from build123d import *

# Parameters (mm, degrees)
BOSS_EXTRUDE1_DEPTH = 0.35
FILLET1_R           = 0.4
FILLET2_R           = 0.5
SKETCH4_W           = 8.5
SKETCH4_H           = 3.36
CUT_EXTRUDE1_DEPTH  = 0.115
SKETCH5_W           = 8.5
SKETCH5_H           = 3.36
CUT_EXTRUDE2_DEPTH  = 0.115
FILLET3_R           = 0.05
SKETCH8_W           = 7.02
SKETCH8_H           = 2.46
BOSS_EXTRUDE2_DEPTH = 0.005
SKETCH9_W           = 7.02
SKETCH9_H           = 2.46
BOSS_EXTRUDE3_DEPTH = 0.005
SKETCH10_W          = 0.5
SKETCH10_H          = 0.12
CUT_EXTRUDE3_DEPTH  = 0.005


with BuildPart() as part:
    # Sketch3 → Boss-Extrude1 (new body)
    with BuildSketch(Plane(origin=(0, 0, 0), x_dir=(1, 0, 0), z_dir=(0, 1, 0))):
        Polygon((-4.25, -4.25), (-3.17, -4.25), (-3.17, -11.79), (5.77, -11.79), (5.77, -7.61), (3.85, -7.61), (3.85, -4.25), (4.25, -4.25), (4.25, 4.25), (-4.25, 4.25), align=None)
    extrude(amount=BOSS_EXTRUDE1_DEPTH)

    # Fillet1
    fillet1_edges = [part.edges().sort_by_distance(p)[0] for p in [
        (5.77, 0.175, 11.79),
        (-3.17, 0.175, 11.79),
        (-3.17, 0.175, 4.25),
        (3.85, 0.175, 4.25),
        (5.77, 0.175, 7.61),
    ]]
    fillet(fillet1_edges, radius=FILLET1_R - 0.0001)  # a hair under: the kernel refuses the full size

    # Fillet2
    fillet2_edges = [part.edges().sort_by_distance(p)[0] for p in [
        (3.85, 0.175, 7.61),
    ]]
    fillet(fillet2_edges, radius=FILLET2_R)

    # Sketch4 → Cut-Extrude1 (cut)
    with BuildSketch(Plane(origin=(0, 0.35, 0), x_dir=(1, 0, 0), z_dir=(0, 1, 0))):
        with Locations((0, -5.93)):
            Rectangle(SKETCH4_W, SKETCH4_H)
    extrude(amount=-CUT_EXTRUDE1_DEPTH, mode=Mode.SUBTRACT)

    # Sketch5 → Cut-Extrude2 (cut)
    with BuildSketch(Plane.XZ):
        with Locations((0, 5.93)):
            Rectangle(SKETCH5_W, SKETCH5_H)
    extrude(amount=-CUT_EXTRUDE2_DEPTH, mode=Mode.SUBTRACT)

    # Fillet3
    fillet3_edges = [part.edges().sort_by_distance(p)[0] for p in [
        (-3.17, 0, 9.50005),
        (0.54, 0, 7.61),
        (4.25, 0, 7.604948974),
        (0, 0, 4.25),
        (-4.25, 0, 0),
        (0, 0, -4.25),
        (4.25, 0, 0),
        (4.86005, 0, 7.61),
        (4.86005, 0.35, 7.61),
        (5.77, 0, 9.7),
        (1.3, 0, 11.79),
        (-3.052872002, 0, 11.672872002),
        (5.652872002, 0, 11.672872002),
        (5.652872002, 0, 7.727127998),
        (5.77, 0.35, 9.7),
        (1.3, 0.35, 11.79),
        (-3.052872002, 0.35, 11.672872002),
        (5.652872002, 0.35, 11.672872002),
        (5.652872002, 0.35, 7.727127998),
        (4.299745519, 0.35, 7.607468077),
        (-3.17, 0.35, 9.50005),
        (0.54, 0.35, 7.61),
        (4.25, 0.35, 7.604948974),
        (4.299745519, 0, 7.607468077),
    ]]
    fillet(fillet3_edges, radius=FILLET3_R)

    # Sketch8 → Boss-Extrude2 (add)
    with BuildSketch(Plane(origin=(0, 0.235, 0), x_dir=(1, 0, 0), z_dir=(0, 1, 0))):
        with Locations((0.34, -5.88)):
            Rectangle(SKETCH8_W, SKETCH8_H)
    extrude(amount=BOSS_EXTRUDE2_DEPTH)

    # Sketch9 → Boss-Extrude3 (add)
    with BuildSketch(Plane.XZ.offset(-0.115)):
        with Locations((0.34, 5.88)):
            Rectangle(SKETCH9_W, SKETCH9_H)
    extrude(amount=BOSS_EXTRUDE3_DEPTH)

    # Sketch10 → Cut-Extrude3 (cut)
    with BuildSketch(Plane.ZY.offset(3.17)):
        with Locations((7.36, 0.175)):
            Rectangle(SKETCH10_W, SKETCH10_H)
    extrude(amount=-CUT_EXTRUDE3_DEPTH, mode=Mode.SUBTRACT)


solid = part.part
Model file for the job. Use its own axes, mm. Coordinates: 2 decimals unless noted, no trailing zeros. Order: outer loops, then holes, each group sorted by start corner. A loop starts at its lowest first (then second) coordinate and runs counter-clockwise, first axis right, second up. Notation, with made-up numbers: M 35.5,-24 L 81.5,-24 A13 ccw 81.5,-6 Z; hole C 43.5,-10.5 d3. An arc over 180 degrees is marked long. Return JSON: item names as keys, results as strings.
1. Saw through at C-C (x = 0.5). Give the cut face in (y, z) (3 decimals), and give its area (3 significant figures).
Ans:
{"outline": "M 0,-4.2 A0.05 ccw 0.05,-4.25 L 0.35,-4.25 L 0.35,4.25 L 0.235,4.25 L 0.235,4.65 L 0.24,4.65 L 0.24,7.11 L 0.235,7.11 L 0.235,7.61 L 0.3,7.61 A0.05 ccw 0.35,7.66 L 0.35,11.74 A0.05 ccw 0.3,11.79 L 0.05,11.79 A0.05 ccw 0,11.74 L 0,7.66 A0.05 ccw 0.05,7.61 L 0.115,7.61 L 0.115,7.11 L 0.11,7.11 L 0.11,4.65 L 0.115,4.65 L 0.115,4.25 L 0.05,4.25 A0.05 ccw 0,4.2 Z", "area": "4.86 mm^2"}
2. Saw through at B-B (z = 10.25). Give the cut face in (x, y).
Ans:
{"outline": "M -3.17,0.05 A0.05 ccw -3.12,0 L 5.72,0 A0.05 ccw 5.77,0.05 L 5.77,0.3 A0.05 ccw 5.72,0.35 L -3.12,0.35 A0.05 ccw -3.17,0.3 Z"}
3. Flat gauge pin, fed straight in: pin 1 (2 mm diameter, centred on x = 0, z = 5.5, fed in from -Y). Where does the tip first touch, or does it go through?
Ans:
{"pin 1": "y = 0.11"}
4. Saw through at D-D (z = 2.5). Give the cut face in (x, y), and give its area (3 significant figures).
Ans:
{"outline": "M -4.25,0.05 A0.05 ccw -4.2,0 L 4.2,0 A0.05 ccw 4.25,0.05 L 4.25,0.35 L -4.25,0.35 Z", "area": "2.97 mm^2"}
5. Drill centre lines: probe 1 along X at (y, z) = (0.1, 8); probe 2 along X at (y, z) = (0.3, -2); probe 3 along Z at (x, y) = (5, 0.1). Where is each one in solid material? Low to high.
Ans:
{"probe 1": "-3.17 to 5.77", "probe 2": "-4.25 to 4.25", "probe 3": "7.61 to 11.79"}
6. Saw through at A-A (x = 4.75). Give the cut face in (y, z), and give its area (3 significant figures).
Ans:
{"outline": "M 0,7.66 A0.05 ccw 0.05,7.61 L 0.3,7.61 A0.05 ccw 0.35,7.66 L 0.35,11.74 A0.05 ccw 0.3,11.79 L 0.05,11.79 A0.05 ccw 0,11.74 Z", "area": "1.46 mm^2"}
